from build123d import *

# Parameters (mm, degrees)
CYLINDER1201_R     = 5
CYLINDER1201_DEPTH = 9.5
CYLINDER1197_R     = 14
CYLINDER1197_DEPTH = 5


with BuildPart() as cylinder1201:
    # Cylinder1201 → Cylinder1201 (new body)
    with BuildSketch(Plane(origin=(462, 85, 142.75), x_dir=(1, 0, 0), z_dir=(0, 0, 1))):
        Circle(CYLINDER1201_R)
    extrude(amount=CYLINDER1201_DEPTH)


with BuildPart() as fusion248002050124:
    # Cylinder1197 → Cylinder1197 (new body)
    with BuildSketch(Plane(origin=(462, 85, 145), x_dir=(1, 0, 0), z_dir=(0, 0, 1))):
        Circle(CYLINDER1197_R)
    extrude(amount=CYLINDER1197_DEPTH)

    # Fusion248002050124: union Cylinder1201
    add(cylinder1201.part)


with BuildPart() as fusion248002050124_1:
    # Fusion248002050124 placement: moved
    add(fusion248002050124.part.moved(Location((0, 0, -32.75))))


solid = fusion248002050124_1.part
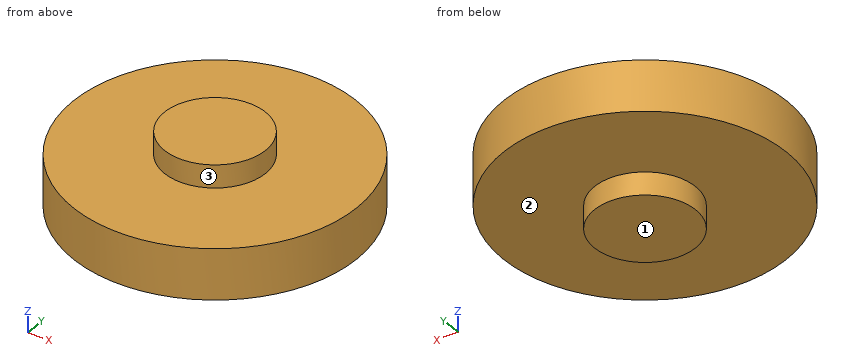
Here's how the part is built. I have some questions about the finished solid (model axes, mm). Face numbers are marked on the shaded views. A direction names the side the tool comes from. Give positions to 0.01 mm unless a question says otherwise; leave off trailing zeros. Loops run counter-clockwise (first coordinate to the right, second up) from the corner with the lowest first, then second, coordinate; pieces in that order, holes last. Notation, with made-up numbers: (52, 33.5) -> (74, 33.5) arc R21 cw to (74, 71.5) -> close; hole circle Ø7 at (84, 28). An arc over 180 degrees is marked (long way). Answer as a JSON object with one key per item and string values. Group by question number.
Item 1: Imagine slicing it at B-B on x = 462. Write out the boundary of the cut face in (y, z).
Item 2: Will these pins go through, and if not, where does the flat tip stop? pin 1 (6 mm diameter, centred on x = 470, y = 82, fed in from -Z); pin 2 (1 mm diameter, centred on y = 77.5, z = 118.5, fed in from +X); pin 3 (8.5 mm diameter, centred on x = 455.5, y = 79.5, fed in from -Z); pin 4 (4 mm diameter, centred on y = 88.5, z = 115.5, fed in from -X).
Item 3: I need wall thicknesses on L1, parallel to Z at x = 465.5, y = 80.5; L2, parallel to Y at x = 462.25, z = 114.25; L3, parallel to Y at x = 461.75, z = 119. Which ranges of each line are inside material? Lowest first, please.
Item 4: On a 3-axis mill with a long thin cutter (end or side, diameter ignored), from which of +Z, -Z, +X, -X, +Y, -Y can I reach the whole of each face in a straight line? I mean the marked faces 1, 2 and 3. Say none if no direction works.
Item 5: Imagine slicing it at D-D on y = 75.75. Write out the boundary of the cut face in (x, z).
Item 6: Imagine slicing it at A-A on y = 85. Write out the boundary of the cut face in (x, z).
Item 7: Imagine slicing it at C-C on x = 452.5. Write out the boundary of the cut face in (y, z), then the cut area to 3 significant figures.
Answer list:
{
 "1": {"outline": "(71, 112.25) -> (80, 112.25) -> (80, 110) -> (90, 110) -> (90, 112.25) -> (99, 112.25) -> (99, 117.25) -> (90, 117.25) -> (90, 119.5) -> (80, 119.5) -> (80, 117.25) -> (71, 117.25) -> close"},
 "2": {"pin 1": "stops at z = 112.25", "pin 2": "passes through", "pin 3": "stops at z = 110", "pin 4": "stops at x = 448.08"},
 "3": {"L1": "z = 112.25 to 117.25", "L2": "y = 71 to 99", "L3": "y = 80.01 to 89.99"},
 "4": {"face 1": "-Z, +X, -X, +Y, -Y", "face 2": "-Z", "face 3": "+Z"},
 "5": {"outline": "(451.49, 112.25) -> (472.51, 112.25) -> (472.51, 117.25) -> (451.49, 117.25) -> close"},
 "6": {"outline": "(448, 112.25) -> (457, 112.25) -> (457, 110) -> (467, 110) -> (467, 112.25) -> (476, 112.25) -> (476, 117.25) -> (467, 117.25) -> (467, 119.5) -> (457, 119.5) -> (457, 117.25) -> (448, 117.25) -> close"},
 "7": {"outline": "(74.72, 112.25) -> (95.28, 112.25) -> (95.28, 117.25) -> (74.72, 117.25) -> close", "area": "103 mm2"}
}
